Read the model definition and answer for the solid it produces. Units are mm, in the model's axes. Face numbers are marked on the shaded views. A direction names the side the tool comes from. Coordinates: 2 decimals unless noted, no trailing zeros. Loops run counter-clockwise (first coordinate to the right, second up) from the corner with the lowest first, then second, coordinate; pieces in that order, holes last.
Q1. Which of the six approach directions +Z, -Z, +X, -X, +Y, -Y give full straight-line access (tool end or side, diameter ignored) to the marked faces 4, 5, 6, 7 and 8?
Q2. Section C-C (x = 13) is taken. Give the vertices of the cut face in (y, z).
Q3. Straight lines are drawn through the part: line 1 (X direction, y = -1.5, z = -11); line 2 (Y direction, x = -17, z = -16.5); line 3 (Y direction, x = 17, z = -17). For each, find the intervals that lie inside material, in ascending order.
Q4. The mould has two halves that part along Z. Classify the marked faces 1, 2 and 3: pulls with the +Z half, pulls with the -Z half, needs draft (parallel to the pull), parting line crosses it, or undercut.
Q5. Section D-D (z = -4) is taken. Give the vertices of the cut face in (x, y).
Q6. Section B-B (x = -7) is taken. Give the vertices of the cut face in (y, z).
Q7. Section A-A (z = -24) is taken. Give the vertices of the cut face in (x, y), then the cut area to 3 significant figures.
Q8. Flat-ended cylindrical pins translate along their axes: P1, Ø1.6, axis at x = -4, z = -11, coming from the +Y side; P2, Ø1.3, axis at y = -16, z = -17.5, coming from the -X side; P3, Ø0.6, axis at x = -19.5, y = -2, coming from the -Z side. Find the tip coordinate at first contact, or state that the pin passes through.
Autodesk Inventor part; units mm, degrees
ref_plane "YZ Plane" through (0, 0, 0) normal (1, 0, 0) x (0, 1, 0)
ref_plane "XZ Plane" through (0, 0, 0) normal (0, 1, 0) x (-1, 0, 0)
ref_plane "XY Plane" through (0, 0, 0) normal (0, 0, 1) x (1, 0, 0)
sketch "スケッチ1" plane through (0, 0, 0) normal (0, 1, 0) x (-1, 0, 0)
  line L0 (-6, -13) -> (6, -13)
  line L1 (6, -13) -> (6, 13)
  line L2 (6, 13) -> (-6, 13)
  line L3 (-6, 13) -> (-6, -13)
  line L4 (-6, -13) -> (6, 13) construction
  line L5 (6, -13) -> (-6, 13) construction
  line L6 (6, 13) -> (-6, 13)
  line L7 (-6, 13) -> (-6, 5)
  line L8 (-6, 5) -> (6, 5)
  line L9 (6, 5) -> (6, 13)
  point P0 (0, 0)
  point P1 (0, 13)
  point P2 (-6, 13)
  point P3 (6, 5)
  dimension "d0" = 12
  dimension "d1" = 26
  dimension "d26" = 12
  dimension "d27" = 8
extrude "押し出し1" add sketch "スケッチ1" against normal blind 3 contours L3 L8 L1 L0
sketch "スケッチ5" plane through (0, 0, 0) normal (1, 0, 0) x (0, 1, 0)
  line L0 (-3, 5) -> (-3, -13)
  line L1 (-3, 5) -> (-3, 13)
  line L2 (-1.6051, 5) -> (-12.6984, 24.2141)
  line L3 (-12.6984, 24.2141) -> (-17.6984, 24.2141)
  line L4 (-16.3866, 0) -> (-3, 0)
  line L5 (0, 5) -> (-3, 5)
  line L6 (-17.6984, 24.2141) -> (-22.1813, 21.6259)
  line L7 (-22.1813, 21.6259) -> (-16.3866, 0)
  line L8 (-12.6984, 24.2141) -> (-8.3683, 26.7141) construction
  line L9 (-8.3683, 26.7141) -> (-7.6183, 25.4151) construction
  circle A0 centre (-7.6183, 25.4151) radius 1 construction
  line L10 (36.5, 48) -> (-6.3683, 23.25) construction
  line L11 (0, 13) -> (36.5, 13) construction
  line L12 (0, -13) -> (0, 5)
  line L13 (-3, 5) -> (-1.6051, 5)
  point P0 (0, 0)
  dimension "d28" = 8
  dimension "d29" = 120
  dimension "d31" = 5
  dimension "d32" = 5
  dimension "d35" = 5
  dimension "d36" = 150
  dimension "d37" = 75
  dimension "d47" = 5
  dimension "d48" = 1.5
  dimension "d49" = 2
  dimension "d50" = 2.5
  dimension "d51" = 49.5
  dimension "d53" = 8
  dimension "d54" = 36.5
  dimension "d55" = 35
extrude "押し出し5" add sketch "スケッチ5" against normal blind 4
sketch "スケッチ6" plane through (-4, 0, 0) normal (-1, 0, 0) x (0, 0, 1)
  line L0 (0, -3) -> (0, -16.3866)
  line L1 (0, -16.3866) -> (21.6259, -22.1813)
  line L2 (21.6259, -22.1813) -> (24.2141, -17.6984)
  line L3 (24.2141, -17.6984) -> (24.2141, -12.6984)
  line L4 (24.2141, -12.6984) -> (5, -1.6051)
  line L5 (0, -3) -> (5, -3)
  line L6 (19.884, -10.1984) -> (14.1259, -20.1716)
  line L7 (24.2141, -12.6984) -> (5.604, -1.9538)
  line L8 (5, -3) -> (5, -1.6051)
  point P0 (0, 0)
  dimension "d38" = 5
extrude "押し出し6" add sketch "スケッチ6" along normal blind 6 contours L6 L4 L3 L2 L1
mirror "ミラー3" about plane through (0, -11.8932, 12.1071) normal (1, 0, 0) of "押し出し5", "押し出し6"
sketch "スケッチ7" plane through (0, 0, 0) normal (0, 1, 0) x (1, 0, 0)
  circle A0 centre (4, -3) radius 1
  circle A1 centre (-4, 11) radius 1
  circle A2 centre (0, 0) radius 0.8
  circle A3 centre (0, 8) radius 0.8
  circle A4 centre (-4, 4) radius 0.8
  circle A5 centre (4, 4) radius 0.8
  circle A6 centre (4, 11) radius 1
  circle A7 centre (-4, -3) radius 1
  line L0 (6, -8) -> (6, -10)
  line L1 (30, -13) -> (9, -13)
  line L2 (33, -9.25) -> (33, -10)
  arc A8 (30, 6.25) -> (30, -6.25) centre (30, 0) ccw
  line L3 (33, 10) -> (33, 9.25)
  line L4 (-30, 13) -> (30, 13)
  line L5 (-33, -10) -> (-33, -9.25)
  arc A9 (-30, -6.25) -> (-30, 6.25) centre (-30, 0) ccw
  line L6 (-33, 9.25) -> (-33, 10)
  line L7 (-9, -13) -> (-30, -13)
  line L8 (-6, -10) -> (-6, -8)
  line L9 (-3, -5) -> (3, -5)
  line L10 (21.75, 7.5) -> (21.75, -7.5)
  line L11 (18.75, -10.5) -> (14, -10.5)
  line L12 (11, -7.5) -> (11, 7.5)
  line L13 (14, 10.5) -> (18.75, 10.5)
  circle A10 centre (9, 10.5) radius 0.85
  circle A11 centre (30, -10.5) radius 0.85
  circle A12 centre (-30, -10.5) radius 0.85
  circle A13 centre (-9, 10.5) radius 0.85
  circle A14 centre (-30, 10.5) radius 0.85
  circle A15 centre (-9, -10.5) radius 0.85
  circle A16 centre (9, -10.5) radius 0.85
  circle A17 centre (30, 10.5) radius 0.85
  line L14 (-11, 7.5) -> (-11, -7.5)
  line L15 (-14, -10.5) -> (-18.75, -10.5)
  line L16 (-21.75, -7.5) -> (-21.75, 7.5)
  line L17 (-18.75, 10.5) -> (-14, 10.5)
  arc A18 (-30, 13) -> (-33, 10) centre (-30, 10) ccw
  arc A19 (-33, 9.25) -> (-30, 6.25) centre (-30, 9.25) ccw
  arc A20 (-30, -6.25) -> (-33, -9.25) centre (-30, -9.25) ccw
  arc A21 (-33, -10) -> (-30, -13) centre (-30, -10) ccw
  arc A22 (-9, -13) -> (-6, -10) centre (-9, -10) ccw
  arc A23 (-3, -5) -> (-6, -8) centre (-3, -8) ccw
  arc A24 (6, -8) -> (3, -5) centre (3, -8) ccw
  arc A25 (6, -10) -> (9, -13) centre (9, -10) ccw
  arc A26 (30, -13) -> (33, -10) centre (30, -10) ccw
  arc A27 (33, -9.25) -> (30, -6.25) centre (30, -9.25) ccw
  arc A28 (30, 6.25) -> (33, 9.25) centre (30, 9.25) ccw
  arc A29 (33, 10) -> (30, 13) centre (30, 10) ccw
  arc A30 (-14, -10.5) -> (-11, -7.5) centre (-14, -7.5) ccw
  arc A31 (-21.75, -7.5) -> (-18.75, -10.5) centre (-18.75, -7.5) ccw
  arc A32 (-18.75, 10.5) -> (-21.75, 7.5) centre (-18.75, 7.5) ccw
  arc A33 (-11, 7.5) -> (-14, 10.5) centre (-14, 7.5) ccw
  arc A34 (18.75, -10.5) -> (21.75, -7.5) centre (18.75, -7.5) ccw
  arc A35 (11, -7.5) -> (14, -10.5) centre (14, -7.5) ccw
  arc A36 (14, 10.5) -> (11, 7.5) centre (14, 7.5) ccw
  arc A37 (21.75, 7.5) -> (18.75, 10.5) centre (18.75, 7.5) ccw
  point P0 (0, 0)
extrude "押し出し7" cut sketch "スケッチ7" against normal up to surface (3 mm away) contours A0 | A1 | A2 | A3 | A4 | A5 | A6 | A7
sketch "スケッチ8" plane through (0, -3, 0) normal (0, -1, 0) x (1, 0, 0)
  line L0 (-6, 5) -> (6, 5)
  line L1 (-6, -13) -> (-6, 5)
  line L2 (6, -13) -> (-6, -13)
  line L3 (6, 5) -> (6, -13)
  point P0 (0, 0)
extrude "押し出し8" add sketch "スケッチ8" along normal blind 23
sketch "スケッチ9" plane through (0, -26, 0) normal (0, -1, 0) x (1, 0, 0)
  circle A0 centre (-4, 3) radius 1
  circle A1 centre (4, 3) radius 1
  circle A2 centre (4, -11) radius 1
  circle A3 centre (4, -11) radius 1
  circle A4 centre (-4, -11) radius 1
  circle A5 centre (-4, -11) radius 1
  point P0 (0, 0)
extrude "押し出し9" cut sketch "スケッチ9" against normal blind 7
sketch "スケッチ10" plane through (10, -17.6984, 24.2141) normal (1, 0, 0) x (0, 0, -1)
  circle A0 centre (2, 2.5) radius 1 construction
  circle A1 centre (7.0529, -1.216) radius 1 construction
  circle A2 centre (2, 2.5) radius 0.8
  circle A3 centre (7.0529, -1.216) radius 0.8
  point P0 (24.2141, 17.6984)
  dimension "d56" = 1.6
  dimension "d57" = 1.6
extrude "押し出し10" cut sketch "スケッチ10" against normal through all
sketch "スケッチ11" plane through (6, 0, 5) normal (1, 0, 0) x (0, 0, -1)
  line L0 (18, 0) -> (18, -26)
  line L1 (18, -11) -> (20, -11)
  line L2 (20, -11) -> (20, -26)
  line L3 (20, -26) -> (18, -26)
  line L4 (18, -26) -> (18, -11)
  line L5 (18, -26) -> (0, -26)
  point P0 (5, 0)
  dimension "d60" = 15
  dimension "d61" = 2
extrude "押し出し11" add sketch "スケッチ11" against normal up to surface (12 mm away)
sketch "スケッチ12" plane through (0, 0, 0) normal (1, 0, 0) x (0, 1, 0)
  line L0 (-26, -15) -> (-11, -15)
  line L1 (-11, -15) -> (-26, -15)
  line L2 (-26, -15) -> (-26, -19)
  line L3 (-26, -19) -> (-11, -19)
  line L4 (-11, -19) -> (-11, -15)
  line L5 (-22, -19) -> (-26, -19)
  line L6 (-26, -19) -> (-26, -37)
  line L7 (-26, -37) -> (-22, -37)
  line L8 (-22, -37) -> (-22, -19)
  line L9 (-26, 5) -> (-26, -15)
  point P0 (0, 0)
  dimension "d64" = 4
  dimension "d65" = 4
  dimension "d66" = 18
extrude "押し出し12" add sketch "スケッチ12" against normal blind 19
mirror "ミラー4" about plane through (0, -18.5, -26) normal (1, 0, 0) of "押し出し12"
sketch "スケッチ13" plane through (-6, -11, -13) normal (0, 1, 0) x (1, 0, 0)
  line L0 (-15, 6) -> (27, 6)
  line L1 (27, 6) -> (27, 2)
  line L2 (27, 2) -> (-15, 2)
  line L3 (-15, 2) -> (-15, 6)
  line L4 (0, 2) -> (-13, 2)
  line L5 (-13, 6) -> (25, 6)
  line L6 (25, 2) -> (25, 6)
  line L7 (-15, 2) -> (-13, 2)
  line L8 (-13, 2) -> (-13, 17)
  line L9 (-13, 17) -> (-15, 17)
  line L10 (-15, 17) -> (-15, 2)
  line L11 (27, 2) -> (25, 2)
  line L12 (25, 2) -> (25, 17)
  line L13 (25, 17) -> (27, 17)
  line L14 (27, 17) -> (27, 2)
  line L15 (-13, 2) -> (-13, 6)
  point P0 (6, -13)
  point P1 (25, 6)
  point P2 (27, 6)
  point P3 (-13, 2)
  point P4 (-15, 6)
  dimension "d75" = 2
  dimension "d76" = 2
  dimension "d77" = 15
extrude "押し出し13" add sketch "スケッチ13" along normal blind 30 contours L10 L9 L8 L0 | L0 L8 L2 L3 | L12 L13 L14 L0 | L0 L1 L2 L6
sketch "スケッチ14" plane through (-6, -11, -13) normal (0, 1, 0) x (1, 0, 0)
  line L0 (0, 2) -> (0, 0)
  line L1 (12, 0) -> (0, 0)
  line L2 (12, 2) -> (12, 0)
  line L3 (12, 2) -> (25, 2)
  line L4 (25, 2) -> (25, 6)
  line L5 (-13, 6) -> (25, 6)
  line L6 (-13, 2) -> (-13, 6)
  line L7 (0, 2) -> (-13, 2)
  point P0 (6, -13)
extrude "押し出し14" add sketch "スケッチ14" along normal blind 5
fillet "フィレット1" radius 10 2 edges at (-19, -6, -17) (19, -6, -17)
sketch "スケッチ16" plane through (21, -11, -15) normal (1, 0, 0) x (0, 0, -1)
  line L0 (15, 30) -> (0, 30)
  line L1 (7.5, 30) -> (15, 17.0096)
  line L2 (15, 0) -> (15, 30)
  point P0 (-15, 11)
  dimension "d85" = 120
extrude "押し出し16" cut sketch "スケッチ16" along normal through all both and the other way through all
sketch "スケッチ17" plane through (19, -26, -37) normal (1, 0, 0) x (0, 0, -1)
  circle A0 centre (-2, 4) radius 1.6
  point P0 (-37, 26)
extrude "押し出し17" cut sketch "スケッチ17" against normal through all
sketch "スケッチ18" plane through (19, -26, -37) normal (1, 0, 0) x (0, 0, -1)
  circle A0 centre (-20, 10) radius 0.8
  circle A1 centre (-20, 2) radius 0.8
  circle A2 centre (-8, 2) radius 0.8
  line L0 (-22, 0) -> (-22, 15)
  line L1 (0, 0) -> (-22, 0)
  point P0 (-37, 26)
  dimension "d90" = 1.6
  dimension "d91" = 1.6
  dimension "d92" = 1.6
  dimension "d93" = 2
  dimension "d94" = 2
  dimension "d95" = 8
  dimension "d96" = 12
extrude "押し出し18" cut sketch "スケッチ18" against normal blind 5
mirror "ミラー5" about plane through (0, 0, 0) normal (1, 0, 0) of "押し出し18"
sketch "スケッチ19" plane through (21, -11, -30) normal (0, 0, -1) x (-1, 0, 0)
  line L0 (0, 0) -> (2, 0)
  line L1 (15, 11) -> (15, 5)
  line L2 (15, 11) -> (15, -15)
  line L3 (15, 0) -> (-20, 0)
  line L4 (-20, 0) -> (-20, 40)
  line L5 (-20, 40) -> (15, 40)
  line L6 (15, 40) -> (15, 0)
  point P0 (21, 11)
extrude "押し出し19" cut sketch "スケッチ19" against normal blind 40
equation "\"d76\" = d75"
properties part number "hipjoint_middle"
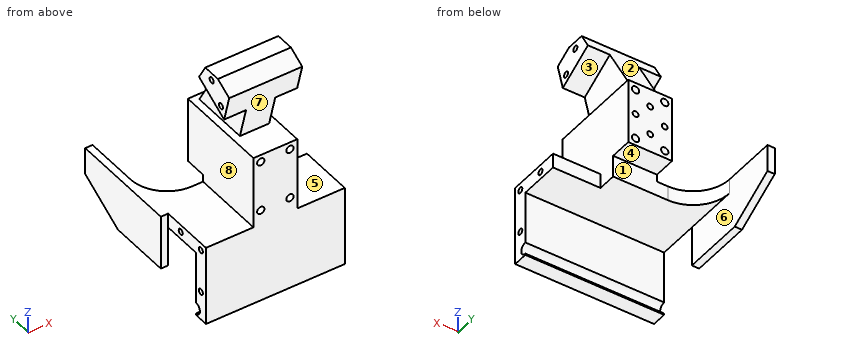
Numbers:
1. face 4: -Z, +X, -X, +Y
1. face 5: +X, +Y, -Y
1. face 6: -Z, +X, +Y
1. face 7: +X, -X, -Y
1. face 8: -X, +Y, -Y
2. outline: (-26, -37) - (-22, -37) - (-22, -36.6) arc R1.6 cw to (-22, -33.4) - (-22, -19) - (-11, -19) - (-11, -15) - (-26, -15) - close
3. line 1: x = -6 to -5, -3 to 3, 5 to 6
3. line 2: y = -26 to -24.62, -23.38 to -16.62, -15.38 to -2
3. line 3: y = -26 to -24.8, -23.2 to -16.8, -15.2 to -11
4. face 1: needs draft
4. face 2: pulls with the +Z half
4. face 3: undercut
5. outline: (-6, -26) - (6, -26) - (6, 0) - (4.8, 0) - (4.8, -3) - (3.2, -3) - (3.2, 0) - (-3.2, 0) - (-3.2, -3) - (-4.8, -3) - (-4.8, 0) - (-6, 0) - close
6. outline: (-26, -37) - (-22, -37) - (-22, -36.6) arc R1.6 cw to (-22, -33.4) - (-22, -19) - (-6, -19) - (-6, -15) - (-26, -15) - close; (-22.18, 21.63) - (-20.17, 14.13) - (-10.2, 19.88) - (-12.7, 24.21) - (-17.7, 24.21) - close; hole circle Ø1.6 at (-18.91, 17.16); hole circle Ø1.6 at (-15.2, 22.21)
7. outline: (-21, -11) - (-19, -11) - (-19, 16.4) - (-21, 16.4) - close; (-19, -26) - (19, -26) - (19, -22) - (-19, -22) - close
7. area: 207 mm2
8. P1: stops at y = -3
8. P2: stops at x = -19
8. P3: stops at z = -30
